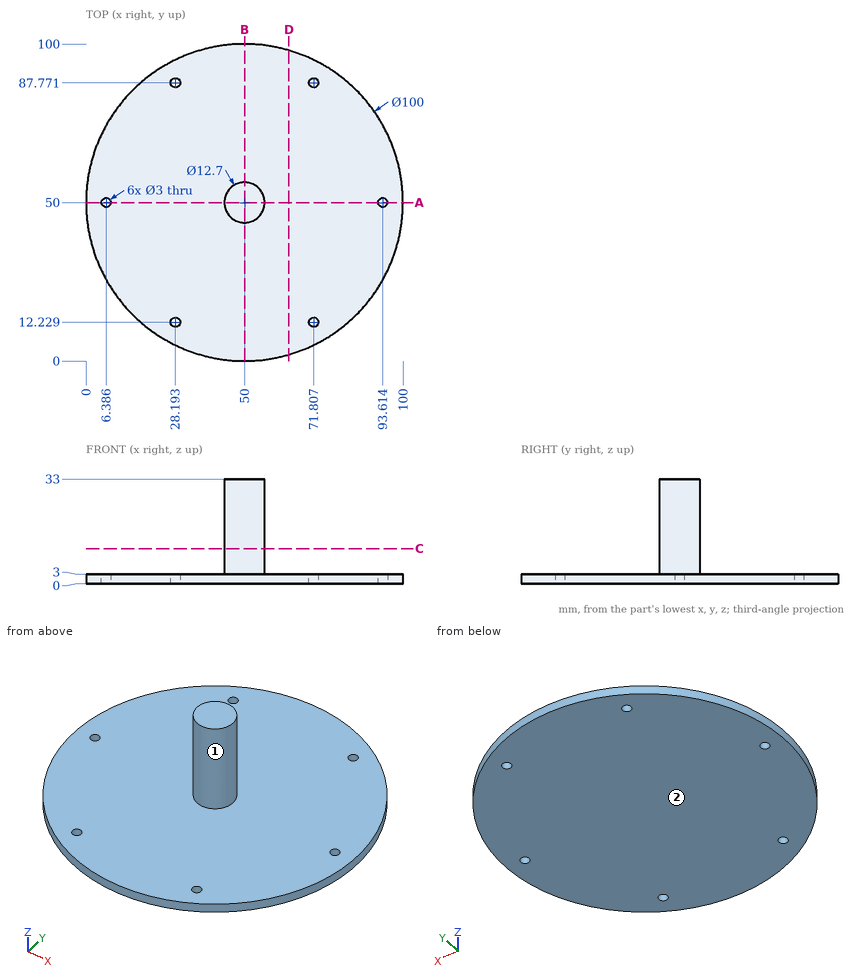
Job drawing, mm, ordinate dimensions from the low corner. One solid piece. A direction names the side the tool comes from. Coordinates: 2 decimals unless noted, no trailing zeros. Order: outer loops, then holes, each group sorted by start corner. A loop starts at its lowest first (then second) coordinate and runs counter-clockwise, first axis right, second up. Notation, with made-up numbers: (-36.75, 4.25) -> (11.25, 4.25) arc R17 cw to (11.25, 14.25) -> close; hole circle Ø5 at (44, 61). An arc over 180 degrees is marked (long way). Put each result on its own line as item: value. Start each with the question number.
(1) Which spindle directions (+Z, -Z, +X, -X, +Y, -Y) get a long thin tool onto all of the face, cutting with end or side? Do the marked faces 1 and 2. Say none if no direction does.
(2) Pin check, flat tips, straight feed: pin 1 Ø5 at (x, y) = (38, 49) entering from +Z; pin 2 Ø1 at (y, z) = (44.5, 22) entering from -X (1 decimal). Stop position of each tip, or through.
(3) Band-saw the part on C-C (z = 11). Give the cut face in (x, y).
(4) Band-saw the part on B-B (x = 50). Give the cut face in (y, z).
(5) Band-saw the part on D-D (x = 64). Give the cut face in (y, z).
(6) Probe line 1 along Z through (x, y) = (74, 11.5); line 2 along X through (y, z) = (52, 5.5); line 3 along Y through (x, z) = (45.5, 5.5). List the from-to ranges inside material, lowest first. Write a range as [from, to].
(7) Band-saw the part on A-A (y = 50). Give the cut face in (x, z), then the cut area to 3 significant figures.
Determined:
1. face 1: +Z
1. face 2: -Z, +X, -X, +Y, -Y
2. pin 1: stops at z = 3
2. pin 2: stops at x = 46.1
3. outline: circle Ø12.7 at (50, 50)
4. outline: (0, 0) -> (100, 0) -> (100, 3) -> (56.35, 3) -> (56.35, 33) -> (43.65, 33) -> (43.65, 3) -> (0, 3) -> close
5. outline: (2, 0) -> (98, 0) -> (98, 3) -> (2, 3) -> close
6. line 1: z = [0, 3]
6. line 2: x = [43.97, 56.03]
6. line 3: y = [45.52, 54.48]
7. outline: (0, 0) -> (4.89, 0) -> (4.89, 3) -> (0, 3) -> close; (7.89, 0) -> (92.11, 0) -> (92.11, 3) -> (56.35, 3) -> (56.35, 33) -> (43.65, 33) -> (43.65, 3) -> (7.89, 3) -> close; (95.11, 0) -> (100, 0) -> (100, 3) -> (95.11, 3) -> close
7. area: 663 mm²
